```python
from build123d import *

# Parameters (mm, degrees)
SZKIC1_R                    = 0.172416741
DODANIE_WYCI_GNI_CIE1_DEPTH = 0.5


with BuildPart() as part:
    # Szkic1 → Dodanie-wyciągnięcie1 (new body)
    with BuildSketch(Plane.XY):
        with BuildLine():
            Line((1.072016687, 2.801924379), (1.072016687, 3.843679809))
            Line((1.072016687, 3.843679809), (0.416833072, 3.843679809))
            Line((0.416833072, 3.843679809), (0.416833072, 2.160150502))
            ThreePointArc((0.416833072, 2.160150502), (0, -2.2), (-0.416833072, 2.160150502))
            Line((-0.416833072, 2.160150502), (-0.416833072, 3.843679809))
            Line((-0.416833072, 3.843679809), (-1.072016687, 3.843679809))
            Line((-1.072016687, 3.843679809), (-1.072016687, 2.801924379))
            ThreePointArc((-1.072016687, 2.801924379), (0, -3), (1.072016687, 2.801924379))
        make_face()
        with Locations((0.74442488, 3.495160541)):
            Circle(SZKIC1_R, mode=Mode.SUBTRACT)
        with Locations((-0.74442488, 3.495160541)):
            Circle(SZKIC1_R, mode=Mode.SUBTRACT)
    extrude(amount=DODANIE_WYCI_GNI_CIE1_DEPTH)


solid = part.part
```
Can you work these out from the model? Positions are in its coordinate system, mm. Coordinates: 2 decimals unless noted, no trailing zeros. Loops run counter-clockwise (first coordinate to the right, second up) from the corner with the lowest first, then second, coordinate; pieces in that order, holes last. Notation, with made-up numbers: (9, 13) -> (35, 13) arc R14 cw to (35, 22) -> close; hole circle Ø1 at (-10, 18.5). An arc over 180 degrees is marked (long way). Put each result on its own line as item: value. Start each with the question number.
Q1. I want a section at C-C (x = -1.5). Write out the boundary of the cut face in (y, z).
Q2. I want a section at D-D (x = 0). Write out the boundary of the cut face in (y, z), plus the area to 3 significant figures.
Q3. I want a section at A-A (y = -2). Write out the boundary of the cut face in (x, z), plus the area to 3 significant figures.
Q4. Thinking about a two-plate mould opening in Y: for faces 1 (the face through (-2, 2, 0)), 2 (the face through (-0.1, -3, 0.2)), 3 (the face through (0.09, -2.2, 0.25)), which applies, pulls with the +Y half, pulls with the -Y half, needs draft (parallel to the pull), parting line crosses it, or undercut?
Q5. I want a section at B-B (z = 0.2). Write out the boundary of the cut face in (x, y), plus the area to 3 significant figures.
Q6. If I drill on line 1 (X direction, y = 3, z = 0.05); line 2 (X direction, y = 0, z = 0.3); line 3 (Y direction, x = -0.75, z = 0.1), over which ranges is the centre line in solid material (lowest first)? Write a range as [from, to].
Q7. I'm going to push flat-ended pins straight in: P1, Ø2, axis at x = -1, y = 1, coming from the -Z side; P2, Ø2.5, axis at x = 0, y = 0, coming from the -Z side. Where does each tip first touch, or does it pass through?
Taken from the geometry:
1. outline: (-2.6, 0) -> (-1.61, 0) -> (-1.61, 0.5) -> (-2.6, 0.5) -> close; (1.61, 0) -> (2.6, 0) -> (2.6, 0.5) -> (1.61, 0.5) -> close
2. outline: (-3, 0) -> (-2.2, 0) -> (-2.2, 0.5) -> (-3, 0.5) -> close
2. area: 0.400 mm2
3. outline: (-2.24, 0) -> (-0.92, 0) -> (-0.92, 0.5) -> (-2.24, 0.5) -> close; (0.92, 0) -> (2.24, 0) -> (2.24, 0.5) -> (0.92, 0.5) -> close
3. area: 1.32 mm2
4. face 1: needs draft
4. face 2: parting line crosses it
4. face 3: undercut
5. outline: (-1.07, 2.8) arc R3 ccw (long way) to (1.07, 2.8) -> (1.07, 3.84) -> (0.42, 3.84) -> (0.42, 2.16) arc R2.2 cw (long way) to (-0.42, 2.16) -> (-0.42, 3.84) -> (-1.07, 3.84) -> close; hole circle Ø0.34 at (-0.74, 3.5); hole circle Ø0.34 at (0.74, 3.5)
5. area: 13.4 mm2
6. line 1: x = [-1.07, -0.42], [0.42, 1.07]
6. line 2: x = [-3, -2.2], [2.2, 3]
6. line 3: y = [-2.9, -2.07], [2.07, 3.32], [3.67, 3.84]
7. P1: stops at z = 0
7. P2: passes through
